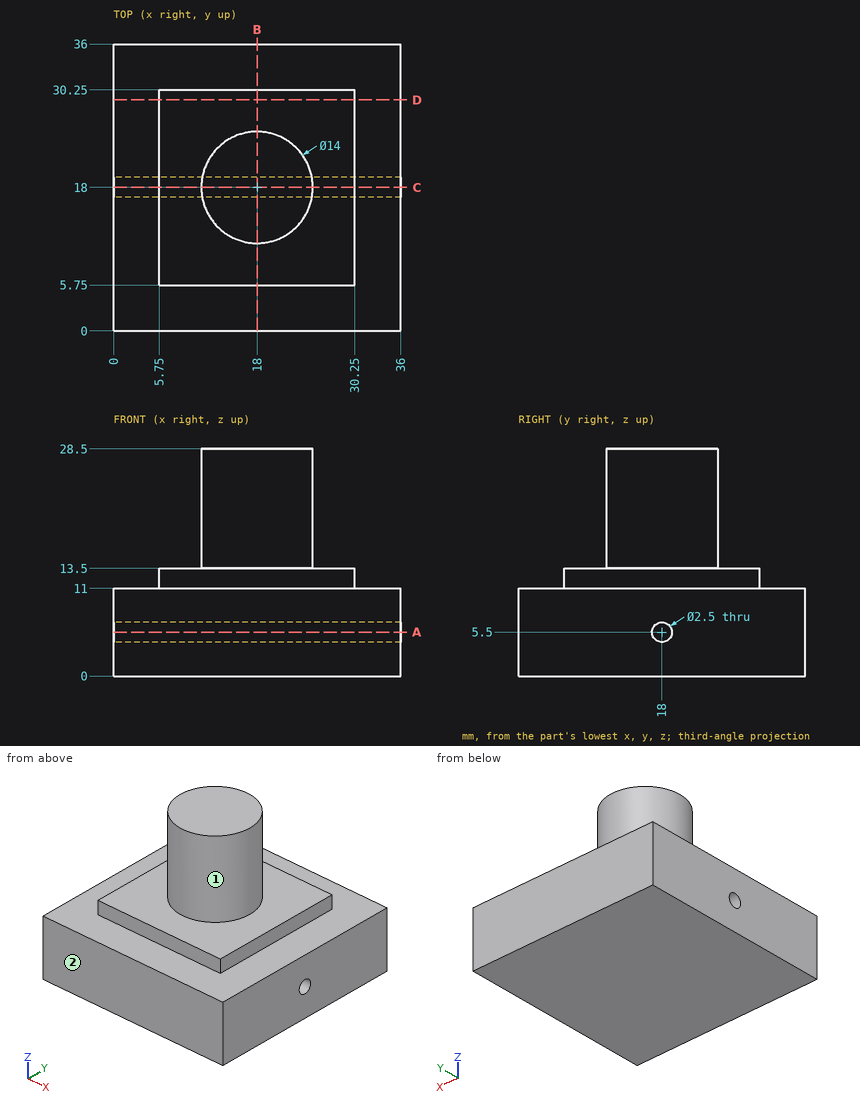
Geometry check sheet. Reference: drawing and pictorial views, mm from the part's lowest x, y, z. A direction names the side the tool comes from. Give positions to 0.01 mm unless a question says otherwise; leave off trailing zeros. Order: outer loops, then holes, each group sorted by start corner. A loop starts at its lowest first (then second) coordinate and runs counter-clockwise, first axis right, second up. Notation, with made-up numbers: M -1.75,3.5 L 32.25,3.5 A14 ccw 32.25,9.5 Z; hole C -12,-38.75 d11. An arc over 180 degrees is marked long. Answer in a Markdown table with one row per item.
1) Cross-section at B-B, the plane x = 18. Enter the section's corners in (y, z).
Filled sheet:
| item | result |
|---|---|
| outline | M 0,0 L 36,0 L 36,11 L 30.25,11 L 30.25,13.5 L 25,13.5 L 25,28.5 L 11,28.5 L 11,13.5 L 5.75,13.5 L 5.75,11 L 0,11 Z; hole C 18,5.5 d2.5 |
2) Access from +Z, -Z, +X, -X, +Y, -Y to the whole of each face (thin tool, end or side, straight path). Record for the marked faces 1 and 2.
Filled sheet:
| item | result |
|---|---|
| face 1 | +Z |
| face 2 | +Z, -Z, +X, -X, -Y |
3) Gauge pin test, flat ends, axial feed: P1, Ø0.8, axis at x = 23, z = 12, coming from the -Y side; P2, Ø5, axis at y = 14, z = 23, coming from the +X side; P3, Ø1.2, axis at y = 12, z = 12.5, coming from the -X side. Record the tip position at first contact, or that the pin passes through.
Filled sheet:
| item | result |
|---|---|
| P1 | stops at y = 5.75 |
| P2 | stops at x = 24.84 |
| P3 | stops at x = 5.75 |
4) Cross-section at A-A, the plane z = 5.5. Enter the section's corners in (x, y), plus the area to 3 significant figures.
Filled sheet:
| item | result |
|---|---|
| outline | M 0,0 L 36,0 L 36,16.75 L 0,16.75 Z; M 0,19.25 L 36,19.25 L 36,36 L 0,36 Z |
| area | 1,210 mm2 |
5) Cross-section at D-D, the plane y = 29. Enter the section's corners in (x, z), plus the area to 3 significant figures.
Filled sheet:
| item | result |
|---|---|
| outline | M 0,0 L 36,0 L 36,11 L 30.25,11 L 30.25,13.5 L 5.75,13.5 L 5.75,11 L 0,11 Z |
| area | 457 mm2 |
6) Cross-section at C-C, the plane y = 18. Enter the section's corners in (x, z), plus the area to 3 significant figures.
Filled sheet:
| item | result |
|---|---|
| outline | M 0,0 L 36,0 L 36,4.25 L 0,4.25 Z; M 0,6.75 L 36,6.75 L 36,11 L 30.25,11 L 30.25,13.5 L 25,13.5 L 25,28.5 L 11,28.5 L 11,13.5 L 5.75,13.5 L 5.75,11 L 0,11 Z |
| area | 577 mm2 |
7) Thickness scan on L1, parallel to Y at x = 28, z = 5.5; L2, parallel to Z at x = 34.5, y = 9; L3, parallel to Z at x = 6, y = 15. Record the ranges inside material, lowest first. Write a range as [from, to].
Filled sheet:
| item | result |
|---|---|
| L1 | y = [0, 16.75], [19.25, 36] |
| L2 | z = [0, 11] |
| L3 | z = [0, 13.5] |
